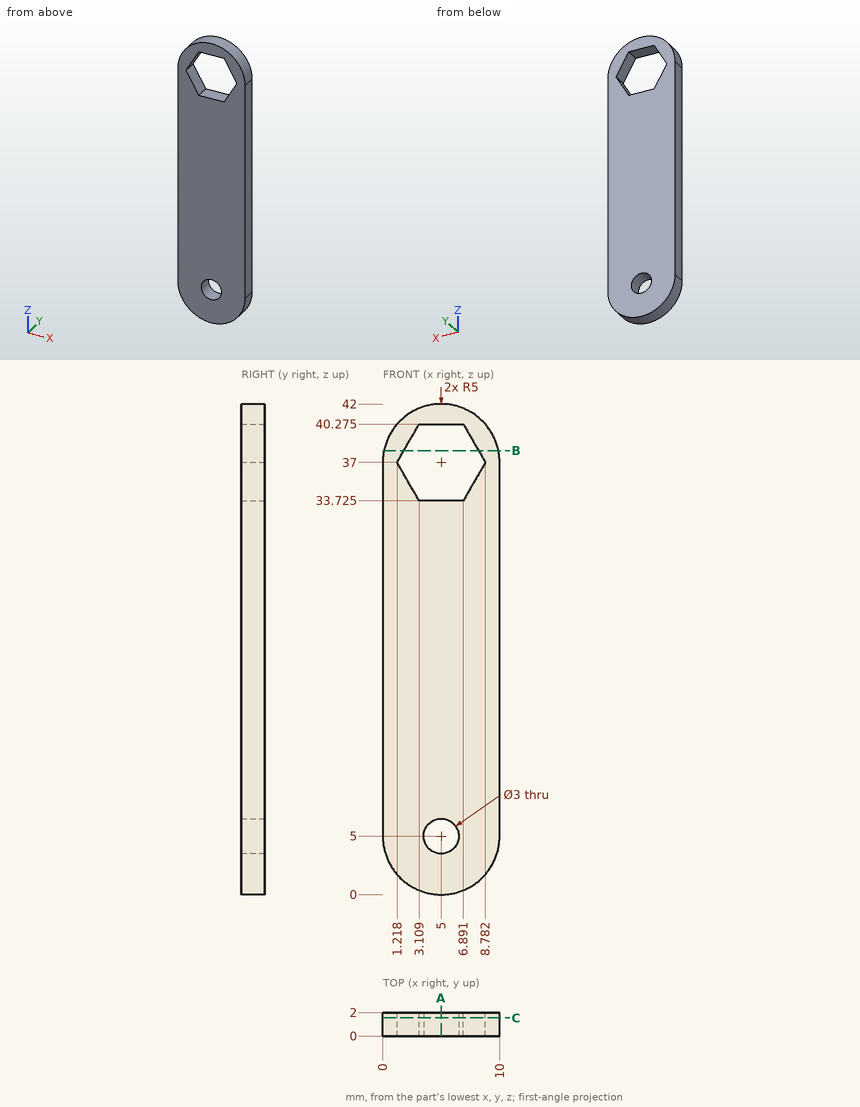
Source: three-view drawing plus pictorial views. Frame: mm from the lowest corner of the part. Round coordinates to 2 decimals unless told otherwise and drop trailing zeros. Write each loop counter-clockwise with the first axis right and the second up, starting at its lowest first coordinate (ties: lowest second). Pieces come first, ordered by that corner, then holes. Notation, with made-up numbers: M -1.75,31.25 L 27.25,31.25 A20 ccw 27.25,51.25 Z; hole C 84.5,-0.5 d1. An arc over 180 degrees is marked long. Use CSV: the item, a comma, the result in double quotes. Start each with the question number.
Q1. Cut plane C-C on y = 1.55. Output: boundary loops of the cut face in (x, z) (1 decimal).
Q2. Cut plane B-B on z = 38. Output: boundary loops of the cut face in (x, y) (1 decimal).
Q3. First-contact query: P1, Ø1.8, axis at x = 5, z = 5, coming from the +Y side. Flat tip, straight axial feed; report the tip coordinate or a pass-through.
Q4. Cut plane A-A on x = 5. Output: boundary loops of the cut face in (y, z) (1 decimal).
Q5. Line query: line 1 (X direction, y = 1.45, z = 5); line 2 (X direction, y = 1.7, z = 37); line 3 (Z direction, x = 3.25, y = 1.35) (1 decimal). Output: solid intervals per line, ascending. Write a range as from..to.
Results found:
1,outline,"M 0,5 A5 ccw 10,5 L 10,37 A5 ccw 0,37 Z; hole M 1.2,37 L 3.1,33.7 L 6.9,33.7 L 8.8,37 L 6.9,40.3 L 3.1,40.3 Z; hole C 5,5 d3"
2,outline,"M 0.1,0 L 1.8,0 L 1.8,2 L 0.1,2 Z; M 8.2,0 L 9.9,0 L 9.9,2 L 8.2,2 Z"
3,P1,"through"
4,outline,"M 0,0 L 2,0 L 2,3.5 L 0,3.5 Z; M 0,6.5 L 2,6.5 L 2,33.7 L 0,33.7 Z; M 0,40.3 L 2,40.3 L 2,42 L 0,42 Z"
5,line 1,"0..3.5, 6.5..10"
5,line 2,"0..1.22, 8.78..10"
5,line 3,"0.3..33.7, 40.3..41.7"
